Work out the finished part from the listing and answer in its coordinate system (mm). A direction names the side the tool comes from. Coordinates: 2 decimals unless noted, no trailing zeros. Loops run counter-clockwise (first coordinate to the right, second up) from the corner with the lowest first, then second, coordinate; pieces in that order, holes last. Notation, with made-up numbers: (80, -15) -> (135, -15) arc R17 cw to (135, 10) -> close; hole circle Ø6 at (22, -8.5). An arc over 180 degrees is marked (long way). Use a Markdown table: item, result.
Autodesk Inventor part; units mm, degrees
ref_plane "YZ Plane" through (0, 0, 0) normal (1, 0, 0) x (0, 1, 0)
ref_plane "XZ Plane" through (0, 0, 0) normal (0, 1, 0) x (-1, 0, 0)
ref_plane "XY Plane" through (0, 0, 0) normal (0, 0, 1) x (1, 0, 0)
sketch "Sketch2" plane through (0, 0, 0) normal (0, 0, 1) x (1, 0, 0)
  arc A0 (-18.496, -13.695) -> (-18.496, 13.695) centre (-16.0813, 0) ccw
  arc A1 (-18.1487, -11.7254) -> (-18.1487, 11.7254) centre (-16.0813, 0) ccw
  line L0 (-16.0813, 0) -> (-18.496, 13.695) construction
  line L1 (-16.0813, 0) -> (-18.496, -13.695) construction
  line L2 (-18.496, 13.695) -> (-18.1487, 11.7254)
  line L3 (-18.496, -13.695) -> (-18.1487, -11.7254)
  line L4 (4.175, 13.9062) -> (4.175, -13.9062)
  line L5 (4.175, 13.9062) -> (-16.0813, 13.9062)
  line L6 (4.175, -13.9062) -> (-16.0812, -13.9063)
  line L7 (-2.175, 13.9062) -> (-2.175, -13.9062) construction
  line L8 (-4.175, 0) -> (4.175, 0) construction
  point P0 (0, 0)
  point P1 (0, 0)
  point P2 (0, 0)
  dimension "d3" = 160
  dimension "d4" = 11.9062
  dimension "d5" = 2
  dimension "d8" = 6.35
extrude "Extrusion1" add sketch "Sketch2" against normal blind 25.4
mirror "Mirror2" about plane through (0, 0, 0) normal (1, 0, 0) of "Extrusion1"
chamfer "Chamfer1" distance 0.25 angle 45 32 edges at (-4.175, 0, 0) (-18.496, -13.695, -12.7) (-18.1487, -11.7254, -12.7) (18.496, -13.695, -12.7) (18.1487, -11.7254, -12.7) (4.175, 0, 0) (18.1487, 11.7254, -12.7) (4.175, 0, -25.4) (-4.175, 0, -25.4) (-18.496, 13.695, -12.7) (-18.1487, 11.7254, -12.7) (0, 13.9062, 0) (-17.2933, 13.8533, 0) (17.2933, 13.8533, 0) (-18.3224, 12.7102, 0) (18.3224, 12.7102, 0) (18.3224, -12.7102, 0) (-17.2933, -13.8533, 0) (0, -13.9063, 0) (17.2933, -13.8533, 0) (-18.3224, -12.7102, 0) (-18.3224, -12.7102, -25.4) (-17.2933, -13.8533, -25.4) (0, -13.9063, -25.4) (17.2933, -13.8533, -25.4) (18.3224, -12.7102, -25.4) (18.3224, 12.7102, -25.4) (18.496, 13.695, -12.7) (0, 13.9062, -25.4) (17.2933, 13.8533, -25.4) (-17.2933, 13.8533, -25.4) (-18.3224, 12.7102, -25.4)
ref_plane "Work Plane3" through (0, 0, 0) normal (1, 0, 0) x (0, 1, 0)
equation "\"d3\" = angle"
equation "\"d5\" = thickness"
equation "\"angle\" = 160deg"
equation "\"thickness\" = 2"
properties part number "two-sided-01"
Q1. Consider line 1 (X direction, y = 0, z = -11); line 2 (Y direction, x = 9, z = -14.5); line 3 (Y direction, x = 7, z = -3.5). Determine where each line is inside the solid, lowest interval first. Write a range as [from, to].
Solved:
| item | result |
|---|---|
| line 1 | [-4.18, 4.18] |
| line 2 | [-13.91, -9.57], [9.57, 13.91] |
| line 3 | [-13.91, -7.7], [7.7, 13.91] |
Q2. Section B-B on y = 0 is taken. Determine the outline of the cut face in (x, z), and give its area (3 significant figures).
Solved:
| item | result |
|---|---|
| outline | (-4.18, -25.15) -> (-3.93, -25.4) -> (3.93, -25.4) -> (4.18, -25.15) -> (4.18, -0.25) -> (3.93, 0) -> (-3.93, 0) -> (-4.18, -0.25) -> close |
| area | 212 mm² |
Q3. Section A-A on z = -21.5 is taken. Determine the outline of the cut face in (x, y), and give its area (3 significant figures).
Solved:
| item | result |
|---|---|
| outline | (-18.45, -13.45) -> (-18.25, -13.74) arc R13.91 ccw to (-16.08, -13.91) -> (0, -13.91) -> (16.08, -13.91) arc R13.91 ccw to (18.25, -13.74) -> (18.45, -13.45) -> (18.19, -11.97) -> (17.9, -11.77) arc R11.91 cw (long way) to (17.9, 11.77) -> (18.19, 11.97) -> (18.45, 13.45) -> (18.25, 13.74) arc R13.91 ccw to (16.08, 13.91) -> (-16.08, 13.91) arc R13.91 ccw to (-18.25, 13.74) -> (-18.45, 13.45) -> (-18.19, 11.97) -> (-17.9, 11.77) arc R11.91 cw (long way) to (-17.9, -11.77) -> (-18.19, -11.97) -> close |
| area | 467 mm² |
Q4. Determine the mould class of faces 1 (the cylindrical face through (-17.184, -13.862, -12.526)), 2 (the flat face through (18.32, -12.7, -12.53)), 3 (the flat face through (0, 0, 0)), 4 (the conical face through (4.05, -0.29, -25.28)) for opening direction X: pulls with the +X half, pulls with the -X half, needs draft (parallel to the pull), parting line crosses it, or undercut.
Solved:
| item | result |
|---|---|
| face 1 | pulls with the -X half |
| face 2 | pulls with the +X half |
| face 3 | needs draft |
| face 4 | undercut |
Q5. Given pin 1 Ø4 at (y, z) = (8.5, -8) entering from -X; pin 2 Ø10 at (y, z) = (7.5, -9.5) entering from +X; pin 3 Ø6 at (y, z) = (6, -9) entering from +X, each flat-ended and moving along its own axis, determine where each tip first touches the part or whether it passes through.
Solved:
| item | result |
|---|---|
| pin 1 | x = -10.47 |
| pin 2 | x = 18.29 |
| pin 3 | x = 8.29 |
Q6. For faces 5 (the flat face through (-18.324, 12.721, -12.526)), 6 (the flat face through (18.32, 12.7, -12.53)), 7 (the conical face through (4.05, 0.29, -0.12)), determine the directions among +Z, -Z, +X, -X, +Y, -Y from which every point of the face is accessible in a straight line to the end or side of a thin tool.
Solved:
| item | result |
|---|---|
| face 5 | +Z, -Z, -X |
| face 6 | +Z, -Z, +X |
| face 7 | +Z |
